```python
from build123d import *

# Parameters (mm, degrees)
SKETCH1_R           = 8.75
BOSS_EXTRUDE1_DEPTH = 6.2
BOSS_EXTRUDE2_DEPTH = 2
FILLET1_R           = 0.8
SKETCH3_R           = 4.75
BOSS_EXTRUDE3_DEPTH = 1.3
SKETCH6_R           = 6.05
BOSS_EXTRUDE5_DEPTH = 1
SKETCH4_R           = 2.35
CUT_EXTRUDE2_DEPTH  = 22.291195363
FILLET2_R           = 2
SKETCH7_R           = 0.9
CUT_EXTRUDE4_DEPTH  = 10


with BuildPart() as part:
    # Sketch1 → Boss-Extrude1 (new body)
    with BuildSketch(Plane(origin=(0, 0, 0), x_dir=(1, 0, 0), z_dir=(0, 1, 0))):
        with Locations(Location((0, 0, 0), (0, 0, 90))):
            Circle(SKETCH1_R)
    extrude(amount=BOSS_EXTRUDE1_DEPTH)

    # Sketch2 → Boss-Extrude2 (add)
    with BuildSketch(Plane.XZ):
        with BuildLine():
            ThreePointArc((7.95, 3.655133376), (8.547660499, 1.870828693), (8.75, 0))
            Line((8.75, 0), (17.45, 0))
            Line((17.45, 0), (17.45, 7.75))
            Line((17.45, 7.75), (7.95, 7.75))
            Line((7.95, 7.75), (7.95, 3.655133376))
        make_face()
        with BuildLine():
            Line((17.45, 0), (8.75, 0))
            ThreePointArc((8.75, 0), (8.547660499, -1.870828693), (7.95, -3.655133376))
            Line((7.95, -3.655133376), (7.95, -7.75))
            Line((7.95, -7.75), (17.45, -7.75))
            Line((17.45, -7.75), (17.45, 0))
        make_face()
    extrude(amount=-BOSS_EXTRUDE2_DEPTH)

    # Fillet1
    fillet1_edges = [part.edges().sort_by_distance(p)[0] for p in [
        (7.95, 1, 3.655133376),
        (7.95, 1, 7.75),
        (17.45, 1, 7.75),
        (17.45, 1, -7.75),
        (7.95, 1, -7.75),
        (7.95, 1, -3.655133376),
    ]]
    fillet(fillet1_edges, radius=FILLET1_R)

    # Sketch3 → Boss-Extrude3 (add)
    with BuildSketch(Plane.XZ):
        with Locations(Location((0, 0, 0), (0, 0, 270))):
            Circle(SKETCH3_R)
    extrude(amount=BOSS_EXTRUDE3_DEPTH)

    # Sketch6 → Boss-Extrude5 (add)
    with BuildSketch(Plane(origin=(0, 6.2, 0), x_dir=(1, 0, 0), z_dir=(0, 1, 0))):
        with Locations(Location((0, 0, 0), (0, 0, 270))):
            Circle(SKETCH6_R)
    extrude(amount=BOSS_EXTRUDE5_DEPTH)

    # Sketch4 → Cut-Extrude2 (cut, through all)
    with BuildSketch(Plane.XZ.offset(1.3)):
        with Locations(Location((0, 0, 0), (0, 0, 270))):
            Circle(SKETCH4_R)
    extrude(amount=-CUT_EXTRUDE2_DEPTH, mode=Mode.SUBTRACT)

    # Fillet2
    # the kernel refuses this fillet: 2 mm, written as the material it takes off along each edge
    with BuildSketch(Plane(origin=(0, 7.2, 0), x_dir=(0, 0, 1), z_dir=(-1, 0, 0))) as fillet2_piece_1:
        with BuildLine():
            CenterArc((4.317949192, -2), FILLET2_R, 30, 60)
            Line((4.317949192, 0), (4.317949192, 0.04))
            Line((4.317949192, 0.04), (6.05, 0.04))
            Line((6.05, 0.04), (6.09, 0))
            ThreePointArc((6.09, 0), (6.09, -0.5), (6.084641016, -0.98))
            Line((6.084641016, -0.98), (6.05, -1))
        make_face()
    revolve(axis=Axis((0, 7.2, 0), (0, 1, 0)), mode=Mode.SUBTRACT)

    # Sketch7 → Cut-Extrude4 (cut)
    with BuildSketch(Plane.XZ):
        with Locations(Location((15.35, -5.25, 0), (0, 0, 270))):
            Circle(SKETCH7_R)
        with Locations(Location((10.15, -5.25, 0), (0, 0, 270))):
            Circle(SKETCH7_R)
        with Locations(Location((12.75, 4.75, 0), (0, 0, 270))):
            Circle(SKETCH7_R)
        with Locations(Location((12.75, 0, 0), (0, 0, 270))):
            Circle(SKETCH7_R)
        with Locations(Location((12.75, -4.75, 0), (0, 0, 270))):
            Circle(SKETCH7_R)
        with Locations(Location((15.35, 5.25, 0), (0, 0, 270))):
            Circle(SKETCH7_R)
        with Locations(Location((15.35, 0, 0), (0, 0, 270))):
            Circle(SKETCH7_R)
        with Locations(Location((10.15, 5.25, 0), (0, 0, 270))):
            Circle(SKETCH7_R)
    extrude(amount=-CUT_EXTRUDE4_DEPTH, mode=Mode.SUBTRACT)


solid = part.part
```
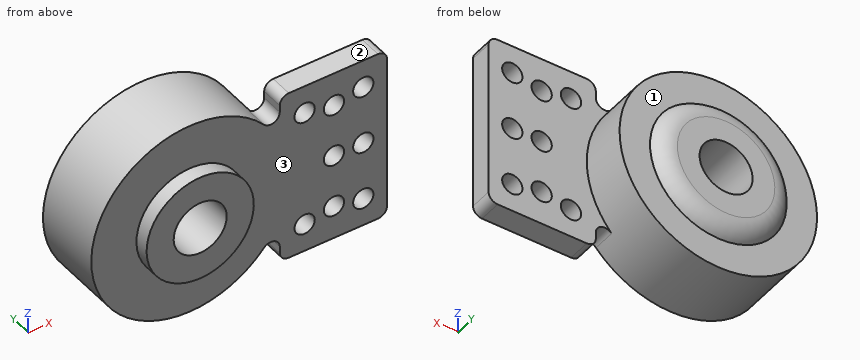
Design review of the part built by this model. Coordinates are the model's own, in mm. Face numbers are marked on the shaded views. A direction names the side the tool comes from. Coordinates: 2 decimals unless noted, no trailing zeros. Order: outer loops, then holes, each group sorted by start corner. A loop starts at its lowest first (then second) coordinate and runs counter-clockwise, first axis right, second up.
1) For the marked faces 1, 2 and 3, list the 3-axis set-ups (+Z, -Z, +X, -X, +Y, -Y) from which the entire face can be reached by the end or side of a thin tool; tool diameter is ignored.
2) Take a section at D-D, the plane z = -5.25. State how many separate pieces and enclosed holes the cut face has, and give its area (3 significant figures).
3) Wall thickness on line 1 along X through (y, z) = (1.15, 0); line 2 along X through (y, z) = (0.85, -5.25); line 3 along Y through (x, z) = (14.75, -6.75): over which ranges is each line inside the solid? List them lowest first.
4) Take a section at B-B, the plane z = 0. Give the boundary of the cut face in (x, y).
5) Take a section at A-A, the plane x = 10.15. Give the boundary of the cut face in (y, z).
6) Take a section at C-C, the plane y = 3. Give the boundary of the cut face in (x, z).
7) Clearance check with flat-ended pins moving along their axes: pin 1 (0.7 mm diameter, centred on y = 1, z = -6.5, fed in from -X); pin 2 (3 mm diameter, centred on x = 10.15, z = -5.25, fed in from -Y); pin 3 (3 mm diameter, centred on x = 10.15, z = 5.25, fed in from +Y). State where each tip first meets the part, or that it passes through.
Returned:
1. face 1: +Y
1. face 2: +Z, +X, +Y, -Y
1. face 3: -Y
2. separate pieces: 4
2. enclosed holes: 0
2. area: 101 mm2
3. line 1: x = -8.75 to -2.35, 2.35 to 11.85, 13.65 to 14.45, 16.25 to 17.45
3. line 2: x = -7 to 9.25, 11.05 to 12, 13.5 to 14.45, 16.25 to 17.45
3. line 3: y = 0 to 2
4. outline: (-8.75, 0) - (-4.75, 0) - (-4.75, -1.3) - (-2.35, -1.3) - (-2.35, 7.2) - (-4.32, 7.2) arc R2 ccw to (-6.05, 6.2) - (-8.75, 6.2) - close; (2.35, -1.3) - (4.75, -1.3) - (4.75, 0) - (11.85, 0) - (11.85, 2) - (8.75, 2) - (8.75, 6.2) - (6.05, 6.2) arc R2 ccw to (4.32, 7.2) - (2.35, 7.2) - close; (13.65, 0) - (14.45, 0) - (14.45, 2) - (13.65, 2) - close; (16.25, 0) - (17.45, 0) - (17.45, 2) - (16.25, 2) - close
5. outline: (0, -7.75) - (2, -7.75) - (2, -6.15) - (0, -6.15) - close; (0, -4.35) - (2, -4.35) - (2, 4.35) - (0, 4.35) - close; (0, 6.15) - (2, 6.15) - (2, 7.75) - (0, 7.75) - close
6. outline: circle Ø17.5 at (0, 0); hole circle Ø4.7 at (0, 0)
7. pin 1: stops at x = -6.22
7. pin 2: stops at y = 0
7. pin 3: stops at y = 2
